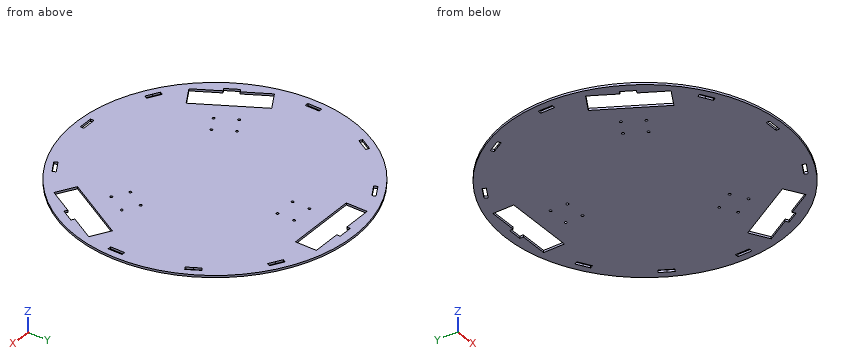
Autodesk Inventor part; units mm, degrees
ref_plane "YZ Plane" through (0, 0, 0) normal (1, 0, 0) x (0, 1, 0)
ref_plane "XZ Plane" through (0, 0, 0) normal (0, 1, 0) x (-1, 0, 0)
ref_plane "XY Plane" through (0, 0, 0) normal (0, 0, 1) x (1, 0, 0)
sketch "Sketch1" plane through (0, 0, 0) normal (0, 0, 1) x (1, 0, 0)
  circle A0 centre (0, 0) radius 200
  line L0 (90.6699, 167.0448) -> (88.1699, 162.7147)
  line L1 (96.8301, 157.7147) -> (99.3301, 162.0448)
  line L2 (162.0448, 99.3301) -> (157.7147, 96.8301)
  line L3 (162.7147, 88.1699) -> (167.0448, 90.6699)
  line L4 (185, 5) -> (190, 5)
  line L5 (190, -5) -> (185, -5)
  line L6 (88.1699, -162.7147) -> (96.8301, -157.7147)
  line L7 (99.3301, -162.0448) -> (90.6699, -167.0448)
  line L8 (-5, -190) -> (-5, -185)
  line L9 (5, -185) -> (5, -190)
  line L10 (-99.3301, -162.0448) -> (-90.6699, -167.0448)
  line L11 (-88.1699, -162.7147) -> (-96.8301, -157.7147)
  line L12 (-190, 5) -> (-190, -5)
  line L13 (-190, -5) -> (-185, -5)
  line L14 (-185, -5) -> (-185, 5)
  line L15 (-167.0448, 90.6699) -> (-162.0448, 99.3301)
  line L16 (-157.7147, 96.8301) -> (-162.7147, 88.1699)
  line L17 (-99.3301, 162.0448) -> (-90.6699, 167.0448)
  line L18 (-88.1699, 162.7147) -> (-96.8301, 157.7147)
  line L19 (-190, -5) -> (-190, 5)
  line L20 (-185, 5) -> (-185, -5)
  line L21 (88.1699, 162.7147) -> (96.8301, 157.7147)
  line L22 (99.3301, 162.0448) -> (90.6699, 167.0448)
  line L23 (162.7147, 88.1699) -> (157.7147, 96.8301)
  line L24 (162.0448, 99.3301) -> (167.0448, 90.6699)
  line L25 (185, 5) -> (185, -5)
  line L26 (190, 5) -> (190, -5)
  line L27 (96.8301, -157.7147) -> (99.3301, -162.0448)
  line L28 (88.1699, -162.7147) -> (90.6699, -167.0448)
  line L29 (-5, -185) -> (5, -185)
  line L30 (-5, -190) -> (5, -190)
  line L31 (-99.3301, -162.0448) -> (-96.8301, -157.7147)
  line L32 (-90.6699, -167.0448) -> (-88.1699, -162.7147)
  line L33 (-190, 5) -> (-185, 5)
  line L34 (-162.0448, 99.3301) -> (-157.7147, 96.8301)
  line L35 (-167.0448, 90.6699) -> (-162.7147, 88.1699)
  line L36 (-99.3301, 162.0448) -> (-96.8301, 157.7147)
  line L37 (-90.6699, 167.0448) -> (-88.1699, 162.7147)
  line L38 (50, 182.5) -> (10, 182.5)
  line L39 (10, 182.5) -> (10, 187.5)
  line L40 (10, 187.5) -> (0, 187.5)
  line L41 (157.7147, 96.8301) -> (162.0448, 99.3301)
  line L42 (167.0448, 90.6699) -> (162.7147, 88.1699)
  line L43 (-99.3301, -162.0448) -> (-96.8301, -157.7147)
  line L44 (-88.1699, -162.7147) -> (-90.6699, -167.0448)
  line L45 (-99.3301, -162.0448) -> (-96.8301, -157.7147)
  line L46 (-88.1699, -162.7147) -> (-90.6699, -167.0448)
  line L47 (-99.3301, -162.0448) -> (-90.6699, -167.0448)
  circle A1 centre (14.945, 125) radius 1.73
  circle A2 centre (14.945, 100.94) radius 1.73
  circle A3 centre (-14.945, 100.94) radius 1.73
  circle A4 centre (-14.945, 125) radius 1.73
  circle A5 centre (-100.7807, -75.4427) radius 1.73
  circle A6 centre (-115.7257, -49.5573) radius 1.73
  circle A7 centre (-79.9441, -63.4127) radius 1.73
  circle A8 centre (-94.8891, -37.5273) radius 1.73
  circle A9 centre (115.7257, -49.5573) radius 1.73
  circle A10 centre (100.7807, -75.4427) radius 1.73
  circle A11 centre (94.8891, -37.5273) radius 1.73
  circle A12 centre (79.9441, -63.4127) radius 1.73
  line L48 (0, 152.5) -> (50, 152.5)
  line L49 (50, 152.5) -> (50, 182.5)
  line L50 (-10, 182.5) -> (-10, 187.5)
  line L51 (-10, 187.5) -> (0, 187.5)
  line L52 (-50, 182.5) -> (-10, 182.5)
  line L53 (0, 152.5) -> (-50, 152.5)
  line L54 (-50, 152.5) -> (-50, 182.5)
  circle A13 centre (0, 0) radius 200
  line L55 (-163.0496, -82.5897) -> (-167.3798, -85.0897)
  line L56 (-167.3798, -85.0897) -> (-162.3798, -93.75)
  line L57 (-183.0496, -47.9487) -> (-163.0496, -82.5897)
  line L58 (-132.0689, -76.25) -> (-157.0689, -32.9487)
  line L59 (-157.0689, -32.9487) -> (-183.0496, -47.9487)
  line L60 (-132.0689, -76.25) -> (-107.0689, -119.5513)
  line L61 (-157.3798, -102.4103) -> (-162.3798, -93.75)
  line L62 (-153.0496, -99.9103) -> (-157.3798, -102.4103)
  line L63 (-133.0496, -134.5513) -> (-153.0496, -99.9103)
  line L64 (-107.0689, -119.5513) -> (-133.0496, -134.5513)
  circle A14 centre (0, 0) radius 200
  line L65 (153.0496, -99.9103) -> (157.3798, -102.4103)
  line L66 (157.3798, -102.4103) -> (162.3798, -93.75)
  line L67 (133.0496, -134.5513) -> (153.0496, -99.9103)
  line L68 (132.0689, -76.25) -> (107.0689, -119.5513)
  line L69 (107.0689, -119.5513) -> (133.0496, -134.5513)
  line L70 (132.0689, -76.25) -> (157.0689, -32.9487)
  line L71 (167.3798, -85.0897) -> (162.3798, -93.75)
  line L72 (163.0496, -82.5897) -> (167.3798, -85.0897)
  line L73 (183.0496, -47.9487) -> (163.0496, -82.5897)
  line L74 (157.0689, -32.9487) -> (183.0496, -47.9487)
  dimension "d6" = 40
  dimension "d8" = 3.46
  dimension "d9" = 360
  dimension "d11" = 50
  dimension "d14" = 360
extrude "Extrusion1" add sketch "Sketch1" along normal blind 3
sketch "Sketch2" plane through (0, 0, 3) normal (0, 0, 1) x (1, 0, 0)
  line L0 (99.3301, 162.0448) -> (96.8301, 157.7147)
  line L1 (99.3301, 162.0448) -> (107.9904, 157.0448)
  line L2 (99.3301, 162.0448) -> (109.3301, 162.0448) construction
  line L3 (107.9904, 157.0448) -> (105.4904, 152.7147)
  line L4 (105.4904, 152.7147) -> (96.8301, 157.7147)
  circle A0 centre (0, 0) radius 200
  line L5 (96.8301, 157.7147) -> (99.3301, 162.0448)
  line L6 (5, 190) -> (15, 190)
  line L7 (5, 190) -> (13.6603, 195) construction
  line L8 (15, 190) -> (15, 185)
  line L9 (15, 185) -> (5, 185)
  line L10 (5, 185) -> (5, 190)
  line L11 (-90.6699, 167.0448) -> (-82.0096, 172.0448)
  line L12 (-90.6699, 167.0448) -> (-85.6699, 175.7051) construction
  line L13 (-82.0096, 172.0448) -> (-79.5096, 167.7147)
  line L14 (-79.5096, 167.7147) -> (-88.1699, 162.7147)
  line L15 (-88.1699, 162.7147) -> (-90.6699, 167.0448)
  line L16 (-162.0448, 99.3301) -> (-157.0448, 107.9904)
  line L17 (-162.0448, 99.3301) -> (-162.0448, 109.3301) construction
  line L18 (-157.0448, 107.9904) -> (-152.7147, 105.4904)
  line L19 (-152.7147, 105.4904) -> (-157.7147, 96.8301)
  line L20 (-157.7147, 96.8301) -> (-162.0448, 99.3301)
  line L21 (-190, 5) -> (-190, 15)
  line L22 (-190, 5) -> (-195, 13.6603) construction
  line L23 (-190, 15) -> (-185, 15)
  line L24 (-185, 15) -> (-185, 5)
  line L25 (-185, 5) -> (-190, 5)
  line L26 (-167.0448, -90.6699) -> (-172.0448, -82.0096)
  line L27 (-167.0448, -90.6699) -> (-175.7051, -85.6699) construction
  line L28 (-172.0448, -82.0096) -> (-167.7147, -79.5096)
  line L29 (-167.7147, -79.5096) -> (-162.7147, -88.1699)
  line L30 (-162.7147, -88.1699) -> (-167.0448, -90.6699)
  line L31 (-99.3301, -162.0448) -> (-107.9904, -157.0448)
  line L32 (-99.3301, -162.0448) -> (-109.3301, -162.0448) construction
  line L33 (-107.9904, -157.0448) -> (-105.4904, -152.7147)
  line L34 (-105.4904, -152.7147) -> (-96.8301, -157.7147)
  line L35 (-96.8301, -157.7147) -> (-99.3301, -162.0448)
  line L36 (-5, -190) -> (-15, -190)
  line L37 (-5, -190) -> (-13.6603, -195) construction
  line L38 (-15, -190) -> (-15, -185)
  line L39 (-15, -185) -> (-5, -185)
  line L40 (-5, -185) -> (-5, -190)
  line L41 (90.6699, -167.0448) -> (82.0096, -172.0448)
  line L42 (90.6699, -167.0448) -> (85.6699, -175.7051) construction
  line L43 (82.0096, -172.0448) -> (79.5096, -167.7147)
  line L44 (79.5096, -167.7147) -> (88.1699, -162.7147)
  line L45 (88.1699, -162.7147) -> (90.6699, -167.0448)
  line L46 (162.0448, -99.3301) -> (157.0448, -107.9904)
  line L47 (162.0448, -99.3301) -> (162.0448, -109.3301) construction
  line L48 (157.0448, -107.9904) -> (152.7147, -105.4904)
  line L49 (152.7147, -105.4904) -> (157.7147, -96.8301)
  line L50 (157.7147, -96.8301) -> (162.0448, -99.3301)
  line L51 (190, -5) -> (190, -15)
  line L52 (190, -5) -> (195, -13.6603) construction
  line L53 (190, -15) -> (185, -15)
  line L54 (185, -15) -> (185, -5)
  line L55 (185, -5) -> (190, -5)
  line L56 (167.0448, 90.6699) -> (172.0448, 82.0096)
  line L57 (167.0448, 90.6699) -> (175.7051, 85.6699) construction
  line L58 (172.0448, 82.0096) -> (167.7147, 79.5096)
  line L59 (167.7147, 79.5096) -> (162.7147, 88.1699)
  line L60 (162.7147, 88.1699) -> (167.0448, 90.6699)
  dimension "d18" = 10
  dimension "d19" = 30
  dimension "d22" = 360
extrude "Extrusion2" cut sketch "Sketch2" against normal blind 10 contours L1 L3 L4 L0 | L11 L13 L14 L15 | L16 L18 L19 L20 | L21 L23 L24 L25 | L31 L33 L34 L35 | L36 L38 L39 L40 | L41 L43 L44 L45 | L51 L53 L54 L55 | L56 L58 L59 L60
properties part number "denew"
Verification items for the finished model (mm, model axes). Round coordinates to 2 decimals unless told otherwise and drop trailing zeros. Order: outer loops, then holes, each group sorted by start corner. A loop starts at its lowest first (then second) coordinate and runs counter-clockwise, first axis right, second up.
1) Material ranges on line 1 (X direction, y = -133.5, z = 1.85); line 2 (X direction, y = -106, z = 1.1); line 3 (X direction, y = 100.94, z = 2.25) (3 decimals), recorded low to high.
Geometry says:
line 1: x = -148.92 to -133.66, -131.23 to 131.23, 133.66 to 148.92
line 2: x = -169.6 to -149.53, -114.89 to 114.89, 149.53 to 169.6
line 3: x = -172.659 to -161.115, -155.342 to -16.675, -13.215 to 13.215, 16.675 to 172.659
2) Depth check by flat-ended pin: pin 1 (4 mm diameter, centred on x = 79.94, y = -63.41, fed in from +Z); pin 2 (0.9 mm diameter, centred on x = 36, z = 2, fed in from -Y); pin 3 (1.5 mm diameter, centred on x = 148.5, z = 1, fed in from +Y); pin 4 (1.5 mm diameter, centred on x = -29, z = 1, fed in from -Y). Enter the tip coordinate at first touch or a pass-through.
Geometry says:
pin 1: stops at z = 3
pin 2: stops at y = -196.82
pin 3: stops at y = 134.8
pin 4: stops at y = -197.99
3) Cross-section at A-A, the plane x = 0. Record the cut outline in (y, z).
Geometry says:
outline: (-200, 0) - (-190, 0) - (-190, 3) - (-200, 3) - close; (-185, 0) - (152.5, 0) - (152.5, 3) - (-185, 3) - close; (187.5, 0) - (200, 0) - (200, 3) - (187.5, 3) - close
4) Cross-section at B-B, the plane y = 140. Record the cut outline in (x, z).
Geometry says:
outline: (-142.83, 0) - (142.83, 0) - (142.83, 3) - (-142.83, 3) - close
5) Cross-section at C-C, the plane z = 1.95. Give the number of separate pieces and of enclosed holes in the cut face, plus the area to 3 significant figures.
Geometry says:
separate pieces: 1
enclosed holes: 24
area: 115,000 mm2
6) Cross-section at D-D, the plane x = -59. Record the cut outline in (y, z), plus the area to 3 significant figures.
Geometry says:
outline: (-191.1, 0) - (191.1, 0) - (191.1, 3) - (-191.1, 3) - close
area: 1,150 mm2
